Work out the finished part from the listing and answer in its coordinate system (mm). A direction names the side the tool comes from. Coordinates: 2 decimals unless noted, no trailing zeros. Loops run counter-clockwise (first coordinate to the right, second up) from the corner with the lowest first, then second, coordinate; pieces in that order, holes last.
```python
from build123d import *

# Parameters (mm, degrees)
F1_DEPTH   = 2.54
F2_C1_SIZE = 1.27
F2_C2_SIZE = 1.2699
F2_C3_SIZE = 1.27
F2_C4_SIZE = 1.2699
F3_SIZE    = 1.26999
F4_W       = 31.75
F4_H       = 19.05
F5_DEPTH   = 2.54
F6_W       = 25.4
F6_H       = 12.7
F7_DEPTH   = 101.6
F8_R       = 6.34999


# Not quite as in the source:
# - a fillet or chamfer is up to 0.001 mm smaller than in the source, because OpenCascade refuses the exact size


with BuildPart() as f1:
    # F0 (on Top) → F1 (new body)
    with BuildSketch(Plane.XY):
        with BuildLine():
            Line((31.75, 0), (0, 0))
            ThreePointArc((0, 0), (8.8381906554, -16.6839242395), (25.5862342852, -25.4))
            Line((25.5862342852, -25.4), (127.1862342852, -25.4))
            Line((127.1862342852, -25.4), (127.1862342852, 0))
            Line((127.1862342852, 0), (50.9862342852, 0))
            Line((50.9862342852, 0), (41.2574698576, -8.163402643))
            ThreePointArc((41.2574698576, -8.163402643), (33.0391135049, -8.1167569468), (31.75, 0))
        make_face()
    extrude(amount=F1_DEPTH)

    # F2: chamfer of 1.27 on 4 edges, made by hand

    # F2_c1
    f2_c1_edges = [f1.edges().sort_by_distance(p)[0] for p in [
        (76.3862342852, -25.4, 0),
    ]]
    chamfer(f2_c1_edges, length=F2_C1_SIZE)

    # F2_c2 (size 1.27 in the source; OpenCascade refuses exactly that, so slightly less here)
    f2_c2_edges = [f1.edges().sort_by_distance(p)[0] for p in [
        (76.3862342852, -25.4, 2.54),
    ]]
    chamfer(f2_c2_edges, length=F2_C2_SIZE)

    # F2_c3
    f2_c3_edges = [f1.edges().sort_by_distance(p)[0] for p in [
        (7.1332744951, -14.8524871452, 0),
    ]]
    chamfer(f2_c3_edges, length=F2_C3_SIZE)

    # F2_c4 (size 1.27 in the source; OpenCascade refuses exactly that, so slightly less here)
    f2_c4_edges = [f1.edges().sort_by_distance(p)[0] for p in [
        (7.133373479, -14.8526022537, 2.54),
    ]]
    chamfer(f2_c4_edges, length=F2_C4_SIZE)

    # F3 (size 1.27 in the source; OpenCascade refuses exactly that, so slightly less here)
    f3_edges = [f1.edges().sort_by_distance(p)[0] for p in [
        (33.039114, -8.116757, 0),
        (33.039114, -8.116757, 2.54),
        (46.121852, -4.081701, 0),
        (46.121852, -4.081701, 2.54),
    ]]
    chamfer(f3_edges, length=F3_SIZE)

    # F4 (on face) → F5 (join)
    with BuildSketch(Plane.YZ.offset(127.1862342852)):
        with Locations((-12.065, 1.27)):
            Rectangle(F4_W, F4_H)
        with BuildLine():
            ThreePointArc((3.81, -8.255), (13.335, 1.27), (3.81, 10.795))
            Line((3.81, 10.795), (3.81, -8.255))
        make_face()
        with BuildLine():
            Line((-27.94, -8.255), (-27.94, 10.795))
            ThreePointArc((-27.94, 10.795), (-37.465, 1.27), (-27.94, -8.255))
        make_face()
    extrude(amount=F5_DEPTH)

    # F6 (on face) → F7 (join)
    with BuildSketch(Plane.YZ.offset(129.7262342852)):
        with Locations((-12.065, 1.27)):
            Rectangle(F6_W, F6_H)
    extrude(amount=F7_DEPTH)

    # F8 (radius 6.35 in the source; OpenCascade refuses exactly that, so slightly less here)
    f8_edges = [f1.edges().sort_by_distance(p)[0] for p in [
        (180.526234, 0.635, 7.62),
        (180.526234, 0.635, -5.08),
        (180.526234, -24.765, -5.08),
        (180.526234, -24.765, 7.62),
        (231.326234, -12.065, 7.62),
        (231.326234, -12.065, -5.08),
    ]]
    fillet(f8_edges, radius=F8_R)


solid = f1.part
```
1. For faces 1 (the flat face through (177, -12, -5.08)), 2 (the flat face through (63, -12, 0)), 3 (the flat face through (129.726, -12, 8)), 4 (the cylindrical face through (181.237, -22.855, -3.269)), determine the directions among +Z, -Z, +X, -X, +Y, -Y from which every point of the face is accessible in a straight line to the end or side of a thin tool.
2. Each of these flat-tipped pins is pushed along its axis until it touches: P1, Ø4, axis at x = 187, y = -9.5, coming from the -Z side; P2, Ø2, axis at x = 38, z = 3, coming from the +Y side; P3, Ø10, axis at x = 175, y = -13.5, coming from the +Z side. Where does it stop, or does it pass through?
3. A cutting plane is placed at C-C, the plane y = -33.5. Give the vertices of the cut face in (x, z), then the cut area to 3 significant figures.
4. Determine the mould class of faces 5 (the cylindrical face through (230.137, -11.887, -2.429)), 6 (the cylindrical face through (128.438, -37.463, 1.479)), 7 (the conical face through (33.01, -8.35, 1.47)) for opening direction Y: released by +Y, released by -Y, zero draft, split by the parting line, or undercut.
5. Straight lines are drawn through the part: probe 1 along Z at (x, y) = (123, -18); probe 2 along X at (y, z) = (-8, 2.5); probe 3 along X at (y, z) = (8, 9.75). For each, find the intervals that lie inside material, in ascending order.
6. A cutting plane is placed at B-B, the plane z = -2. Give the vertices of the cut face in (x, y), then the cut area to 3 significant figures.
Answers below:
1. face 1: -Z, +X, +Y, -Y
1. face 2: -Z, -X, +Y, -Y
1. face 3: +Z, +X
1. face 4: -Z, +X, -Y
2. P1: stops at z = -5.08
2. P2: stops at y = -10.32
2. P3: stops at z = 7.62
3. outline: (127.19, -6.46) - (129.73, -6.46) - (129.73, 9) - (127.19, 9) - close
3. area: 39.3 mm2
4. face 5: zero draft
4. face 6: released by -Y
4. face 7: undercut
5. probe 1: z = 0 to 2.54
5. probe 2: x = 4.01 to 31.23, 43.37 to 231.21
5. probe 3: x = 127.19 to 129.73
6. outline: (127.19, -36.89) - (129.73, -36.89) - (129.73, -23.86) - (230.42, -23.86) - (230.42, -0.27) - (129.73, -0.27) - (129.73, 12.76) - (127.19, 12.76) - close
6. area: 2,500 mm2
